Read the model definition and answer for the solid it produces. Units are mm, in the model's axes. Face numbers are marked on the shaded views. A direction names the side the tool comes from. Round coordinates to 2 decimals unless told otherwise and drop trailing zeros. Write each loop counter-clockwise with the first axis right and the second up, starting at its lowest first coordinate (ties: lowest second). Pieces come first, ordered by that corner, then holes. Notation, with made-up numbers: (23, -39) - (57, -39) arc R30 ccw to (57, -12) - close; hole circle Ø6 at (-38.75, 77). An arc over 180 degrees is marked (long way). Answer as CSV lines item,"result". Start each with the question number.
1) Each of these flat-tipped pins is pushed along its axis until it touches: pin 1 (12 mm diameter, centred on y = 15, z = 32.5, fed in from -X); pin 2 (1.5 mm diameter, centred on x = 22, z = 4.5, fed in from +Y); pin 3 (1.5 mm diameter, centred on x = 52, y = 17, fed in from -Z); pin 4 (8.5 mm diameter, centred on x = 6.5, z = 22.5, fed in from -Y). Where does it stop, or does it pass through?
2) Find section C-C on y = 21. Determine the outline of the cut face in (x, z), then the cut area to 3 significant figures.
3) Find section B-B on x = 30. Determine the outline of the cut face in (y, z), then the cut area to 3 significant figures.
4) Which of the six approach directions +Z, -Z, +X, -X, +Y, -Y give full straight-line access (tool end or side, diameter ignored) to the marked faces 1, 2 and 3?
5) Consider line 1 along X through (y, z) = (18, 24); line 2 along Z through (x, y) = (7, 15); line 3 along X through (y, z) = (14.5, 7). Determine where each line is inside the solid, lowest interval first.
6) For a pull along Y with two mould halves and no side action, classify the marked faces 4, 5, 6 and 7 as +Y half, -Y half, draft (parallel to the pull), parting line (faces both ways), or undercut.
7) Find section A-A on z = 15. Determine the outline of the cut face in (x, y).
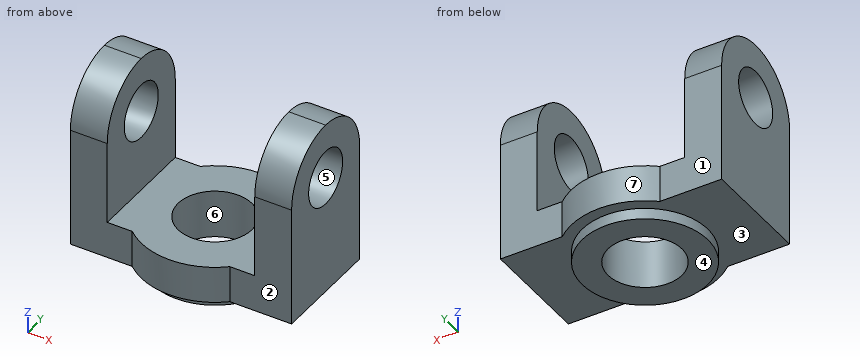
from build123d import *

# Parameters (mm, degrees)
F1_DEPTH  = 47.5
F2_W      = 40
F2_H      = 37.5
F3_DEPTH  = 205
F4_W      = 26.4575131106
F4_H      = 37.5
F5_DEPTH  = 25
F6_R      = 17
F7_DEPTH  = 3
F8_R      = 10
F9_DEPTH  = 25
F11_DEPTH = 125
F12_R     = 14.99999


# Not quite as in the source:
# - a fillet or chamfer is up to 0.001 mm smaller than in the source, because OpenCascade refuses the exact size


with BuildPart() as f1:
    # F0 (on Top) → F1 (new body)
    with BuildSketch(Plane.XY):
        Polygon((0, 15), (0, 0), (16.7712434447, 0), (43.2287565553, 0), (60, 0), (60, 15), (60, 30), (43.2287565553, 30), (16.7712434447, 30), (0, 30), align=None)
        with BuildLine():
            Line((49.2664991614, 20.3667504193), (60, 15))
            Line((60, 15), (50, 15))
            ThreePointArc((50, 15), (49.8157763314, 17.7083220609), (49.2664991614, 20.3667504193))
        make_face(mode=Mode.SUBTRACT)
        with BuildLine():
            Line((43.2287565553, 0), (16.7712434447, 0))
            ThreePointArc((16.7712434447, 0), (30, -5), (43.2287565553, 0))
        make_face()
        with BuildLine():
            ThreePointArc((43.2287565553, 30), (30, 35), (16.7712434447, 30))
            Line((16.7712434447, 30), (43.2287565553, 30))
        make_face()
        with BuildLine():
            Line((50, 15), (60, 15))
            Line((60, 15), (49.2664991614, 20.3667504193))
            ThreePointArc((49.2664991614, 20.3667504193), (49.8157763314, 17.7083220609), (50, 15))
        make_face()
    extrude(amount=F1_DEPTH)

    # F2 (on face) → F3 (cut)
    with BuildSketch(Plane.XZ):
        with Locations((30, 28.75)):
            Rectangle(F2_W, F2_H)
    extrude(amount=-F3_DEPTH, mode=Mode.SUBTRACT)

    # F4 (on face) → F5 (cut)
    with BuildSketch(Plane(origin=(0, 0, 0), x_dir=(-1, 0, 0), z_dir=(0, 1, 0))):
        with Locations((-30, 28.75)):
            Rectangle(F4_W, F4_H)
    extrude(amount=-F5_DEPTH, mode=Mode.SUBTRACT)

    # F6 (on face) → F7 (join)
    with BuildSketch(Plane(origin=(0, 0, 0), x_dir=(1, 0, 0), z_dir=(0, 0, -1))):
        with Locations((30, -15)):
            Circle(F6_R)
    extrude(amount=F7_DEPTH)

    # F8 (on face) → F9 (cut)
    with BuildSketch(Plane(origin=(0, 0, -3), x_dir=(1, 0, 0), z_dir=(0, 0, -1))):
        with Locations((30, -15)):
            Circle(F8_R)
    extrude(amount=-F9_DEPTH, mode=Mode.SUBTRACT)

    # F10 (on face) → F11 (cut)
    with BuildSketch(Plane.YZ.offset(60)):
        with BuildLine():
            ThreePointArc((15, 25), (20.3033008589, 27.1966991411), (22.5, 32.5))
            ThreePointArc((22.5, 32.5), (9.6966991411, 37.8033008589), (15, 25))
        make_face()
    extrude(amount=-F11_DEPTH, mode=Mode.SUBTRACT)

    # F12 (radius 15 in the source; OpenCascade refuses exactly that, so slightly less here)
    f12_edges = [f1.edges().sort_by_distance(p)[0] for p in [
        (55, 0, 47.5),
        (55, 30, 47.5),
        (5, 0, 47.5),
        (5, 30, 47.5),
    ]]
    fillet(f12_edges, radius=F12_R)


solid = f1.part
Check values:
1,pin 1,"passes through"
1,pin 2,"stops at y = 33.64"
1,pin 3,"stops at z = 0"
1,pin 4,"stops at y = 0"
2,outline,"(0, 0) - (14.09, 0) - (14.09, -3) - (22, -3) - (22, 10) - (10, 10) - (10, 28) - (0, 28) - close; (0, 37) - (10, 37) - (10, 46.25) - (0, 46.25) - close; (38, -3) - (45.91, -3) - (45.91, 0) - (60, 0) - (60, 28) - (50, 28) - (50, 10) - (38, 10) - close; (50, 37) - (60, 37) - (60, 46.25) - (50, 46.25) - close"
2,area,"1,030 mm^2"
3,outline,"(-5, 0) - (-2, 0) - (-2, -3) - (5, -3) - (5, 10) - (-5, 10) - close; (25, -3) - (32, -3) - (32, 0) - (35, 0) - (35, 10) - (25, 10) - close"
3,area,"242 mm^2"
4,face 1,"+Z, -Z, -X, +Y"
4,face 2,"+Z, -Z, +X, -Y"
4,face 3,"-Z"
5,line 1,"x = 0 to 10, 50 to 60"
5,line 2,"z = 0 to 25, 40 to 47.5"
5,line 3,"x = 0 to 20.01, 39.99 to 60"
6,face 4,"draft"
6,face 5,"undercut"
6,face 6,"undercut"
6,face 7,"+Y half"
7,outline,"(0, 0) - (10, 0) - (10, 30) - (0, 30) - close; (50, 0) - (60, 0) - (60, 30) - (50, 30) - close"
